Geometry: final body of the model. Coordinates: model frame, mm. Face numbers are marked on the shaded views. A direction names the side the tool comes from. Give positions to 0.01 mm unless a question says otherwise; leave off trailing zeros. Write each loop counter-clockwise with the first axis right and the second up, starting at its lowest first coordinate (ties: lowest second). Pieces come first, ordered by that corner, then holes.
Q1. Cut plane C-C on z = 9.5. Return the cut outline in (x, y).
Q2. Reachability of the marked faces 4 and 5 from +Z, -Z, +X, -X, +Y, -Y: full face, straight path, thin tool, end or side. Return the list, or none.
Q3. Cut plane D-D on y = 8.5. Return the cut outline in (x, z), plus the area to 3 significant figures.
Q4. Cut plane A-A on x = 8. Return the cut outline in (y, z), plus the area to 3 significant figures.
Q5. Draft query along Y for the marked faces 1, 2 and 3. Return one class per face: pulls with the +Y half, pulls with the -Y half, needs draft (parallel to the pull), parting line crosses it, or undercut.
Q6. Line query: L1, parallel to Z at x = -6, y = 3; L2, parallel to Y at x = -6.75, z = 5; L3, parallel to Y at x = 0, z = 9.3. Output: solid intervals per line, ascending.
Q7. Cut plane B-B on z = 2.5. Return the cut outline in (x, y), plus the area to 3 significant figures.
Q8. Pin query (flat end, axial travel): pin 1 (1.5 mm diameter, centred on y = 3.5, z = 9.5, fed in from -X); pin 2 (3 mm diameter, centred on x = -8.45, y = 0, fed in from -Z); pin 3 (6 mm diameter, centred on x = -6.5, z = 4.5, fed in from +Y); pin 4 (4 mm diameter, centred on x = 8.5, y = -0.5, fed in from +Z). Return the tip coordinate at first contact, or that it passes through.
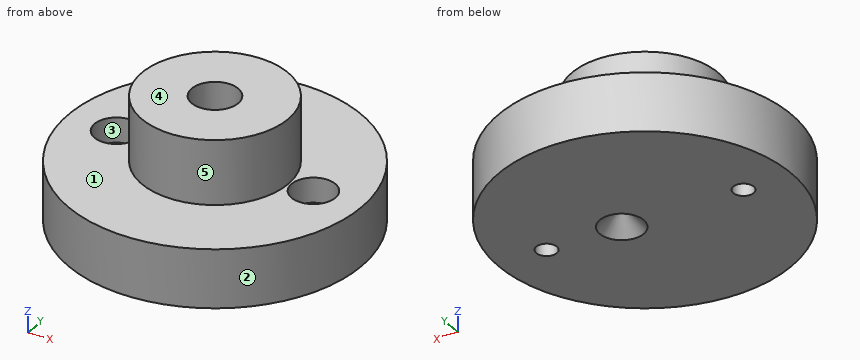
```python
from build123d import *

# Parameters (mm, degrees)
SKETCH1_R                  = 12.7
BOSS_EXTRUDE1_DEPTH        = 5.08
SKETCH3_R                  = 6.35
BOSS_EXTRUDE2_DEPTH        = 5.588
SKETCH5_R                  = 2.0193
CUT_EXTRUDE1_DEPTH         = 5.588
F_50_0_07_DIAMETER_HOLE1_D = 1.778
SKETCH6_R                  = 1.905
CUT_EXTRUDE2_DEPTH         = 2.159


with BuildPart() as part:
    # Sketch1 → Boss-Extrude1 (new body)
    with BuildSketch(Plane.XY):
        Circle(SKETCH1_R)
    extrude(amount=BOSS_EXTRUDE1_DEPTH)

    # Sketch3 → Boss-Extrude2 (add)
    with BuildSketch(Plane.XY.offset(5.08)):
        Circle(SKETCH3_R)
    extrude(amount=BOSS_EXTRUDE2_DEPTH)

    # Sketch5 → Cut-Extrude1 (cut)
    with BuildSketch(Plane.XY.offset(10.668)):
        Circle(SKETCH5_R)
    extrude(amount=-CUT_EXTRUDE1_DEPTH, mode=Mode.SUBTRACT)

    # #50 (0.07) Diameter Hole1 (through all)
    with Locations(Plane.XY.offset(5.08)):
        with Locations((-8.45058, 0), (8.45058, 0)):
            Hole(F_50_0_07_DIAMETER_HOLE1_D / 2)

    # Sketch6 → Cut-Extrude2 (cut)
    with BuildSketch(Plane.XY.offset(5.08)):
        with Locations((-8.45058, 0)):
            Circle(SKETCH6_R)
        with Locations((8.45058, 0)):
            Circle(SKETCH6_R)
    extrude(amount=-CUT_EXTRUDE2_DEPTH, mode=Mode.SUBTRACT)

    # Cut-Extrude3 cone 1 section (through the dimple's axis) → Cut-Extrude3 (revolve, cut)
    with BuildSketch(Plane.YZ.offset(1.99898)):
        Polygon((0, 0), (1.905, 0), (0, 1.905), align=None)
    revolve(axis=Axis((1.99898, 0, 0), (0, 0, 1)), mode=Mode.SUBTRACT)


solid = part.part
```
Data:
1. outline: circle Ø12.7 at (0, 0); hole circle Ø4.04 at (0, 0)
2. face 4: +Z, +X, -X, +Y, -Y
2. face 5: +Z
3. outline: (-9.44, 0) - (9.44, 0) - (9.44, 5.08) - (-9.44, 5.08) - close
3. area: 95.9 mm2
4. outline: (-9.86, 0) - (-0.77, 0) - (-0.77, 2.92) - (-1.85, 2.92) - (-1.85, 5.08) - (-9.86, 5.08) - close; (0.77, 0) - (9.86, 0) - (9.86, 5.08) - (1.85, 5.08) - (1.85, 2.92) - (0.77, 2.92) - close
4. area: 87.7 mm2
5. face 1: needs draft
5. face 2: parting line crosses it
5. face 3: undercut
6. L1: z = 0 to 5.08
6. L2: y = -10.76 to -0.86, 0.86 to 10.76
6. L3: y = -6.35 to -2.02, 2.02 to 6.35
7. outline: circle Ø25.4 at (0, 0); hole circle Ø1.78 at (-8.45, 0); hole circle Ø1.78 at (8.45, 0)
7. area: 502 mm2
8. pin 1: stops at x = -5.72
8. pin 2: stops at z = 0
8. pin 3: stops at y = 12.21
8. pin 4: stops at z = 5.08
